Input: part model. Units: mm. Frame: model coordinates. A direction names the side the tool comes from. Give positions to 0.01 mm unless a question says otherwise; leave off trailing zeros. Loops run counter-clockwise (first coordinate to the right, second up) from the corner with the lowest first, then second, coordinate; pieces in that order, holes last. Notation, with made-up numbers: M -15,3 L 25,3 A20 cw 25,7 Z; hole C 47,22.25 d8. An arc over 180 degrees is marked long. Answer as a JSON object with one key per item and string values. Group by question number.
1) Section query B-B on x = -4.5. Return loops of the section in (y, z), plus the area to 3 significant figures.
2) Draft query along Y for faces 3 (the flat face through (0, 1, 1)), 4 (the flat face through (4.82, 6.5, 0.49)), 5 (the flat face through (-6.2, 0.9, 0.7)). Return one class per face: +Y half, -Y half, draft (parallel to the pull), parting line (faces both ways), or undercut.
3) Section query A-A on y = 6. Return loops of the section in (x, z).
4) Section query D-D on x = -2.5. Return loops of the section in (y, z).
5) Ray query, L1, parallel to Y at x = 1, z = 0.95; L2, parallel to Y at x = -3.25, z = 0.6; L3, parallel to X at y = -3.5, z = 0.7. Return the intervals inside material, ascending.
6) Access query for faces 1 (the flat face through (-4.689, 6.593, 0.493)), 2 (the flat face through (-4, 5, 0.5)). Directions: +Z, -Z, +X, -X, +Y, -Y. A direction counts if a zero-diameter tool reaches every point of the face in a straight line with its end or side. Return the directions, or none.
7) Section query C-C on z = 0.2. Return loops of the section in (x, y).
8) First-contact query: P1, Ø2, axis at x = 2.5, y = 0, coming from the -Z side; P2, Ø2, axis at x = -3.5, y = 4, coming from the +Z side; P3, Ø0.6, axis at x = 2, z = 0.5, coming from the +Y side. Flat tips, straight axial feed; report the tip coordinate or a pass-through.
from build123d import *

# Parameters (mm, degrees)
PAD_DEPTH    = 1
POCKET_DEPTH = 0.5
PAD001_DEPTH = 0.5


with BuildPart() as part:
    # Sketch → Pad (new body)
    with BuildSketch(Plane.XY):
        Polygon((0, 10), (-9.510565, 3.09017), (-5.877853, -8.09017), (5.877853, -8.09017), (9.510565, 3.09017), align=None)
    extrude(amount=PAD_DEPTH)

    # Sketch001 (on Face7 of Pad) → Pocket (cut)
    with BuildSketch(Plane.XY.offset(1)):
        Polygon((0, 9.5), (-9.035037, 2.935661), (-5.58396, -7.685661), (5.58396, -7.685661), (9.035037, 2.935661), align=None)
    extrude(amount=-POCKET_DEPTH, mode=Mode.SUBTRACT)

    # Sketch002 (on Face13 of Pocket) → Pad001 (join)
    with BuildSketch(Plane.XY.offset(0.5)):
        Polygon((-9.035037, 2.935661), (-2.75, 2.935661), (0, 9.5), (2.75, 2.935661), (9.035037, 2.935661), (3.5, -1.035616), (5.58396, -7.685661), (0, -3.9), (-5.58396, -7.685661), (-3.5, -1.035616), align=None)
    extrude(amount=PAD001_DEPTH)


solid = part.part
Output:
{
 "1": {"outline": "M -8.09,0 L 6.73,0 L 6.73,1 L 6.23,1 L 6.23,0.5 L 2.94,0.5 L 2.94,1 L -0.32,1 L -0.32,0.5 L -4.23,0.5 L -4.23,1 L -6.95,1 L -6.95,0.5 L -7.69,0.5 L -7.69,1 L -8.09,1 Z", "area": "10.9 mm^2"},
 "2": {"face 3": "draft", "face 4": "+Y half", "face 5": "undercut"},
 "3": {"outline": "M -5.51,0 L 5.51,0 L 5.51,1 L 4.82,1 L 4.82,0.5 L 1.47,0.5 L 1.47,1 L -1.47,1 L -1.47,0.5 L -4.82,0.5 L -4.82,1 L -5.51,1 Z"},
 "4": {"outline": "M -8.09,0 L 8.18,0 L 8.18,1 L 7.68,1 L 7.68,0.5 L 3.53,0.5 L 3.53,1 L -5.59,1 L -5.59,0.5 L -7.69,0.5 L -7.69,1 L -8.09,1 Z"},
 "5": {"L1": "y = -8.09 to -7.69, -4.58 to 7.11, 8.77 to 9.27", "L2": "y = -8.09 to -7.69, -6.1 to 2.94, 7.14 to 7.64", "L3": "x = -7.37 to -6.94, -4.27 to 4.27, 6.94 to 7.37"},
 "6": {"face 1": "+Z, -Z, -X, +Y", "face 2": "+Z"},
 "7": {"outline": "M -9.51,3.09 L -5.88,-8.09 L 5.88,-8.09 L 9.51,3.09 L 0,10 Z"},
 "8": {"P1": "stops at z = 0", "P2": "stops at z = 0.5", "P3": "stops at y = 8.76"}
}
